Model file for the job. Use its own axes, mm. Round coordinates to 2 decimals unless told otherwise and drop trailing zeros. Order: outer loops, then holes, each group sorted by start corner. A loop starts at its lowest first (then second) coordinate and runs counter-clockwise, first axis right, second up. Notation, with made-up numbers: (-24.5, 2) -> (0.5, 2) arc R12 cw to (0.5, 7) -> close; hole circle Ø2 at (37, 63.5). An arc over 180 degrees is marked (long way). Put each result on its own line as item: value. Start each with the question number.
Q1. Cut at C-C, the plane y = -0.2. List the corners of the cut face in (x, z), and give its area (3 significant figures).
Q2. Flat gauge pins, fed straight in: P1, Ø1, axis at x = 1, y = 0.5, coming from the +Z side; P2, Ø1, axis at y = -0.5, z = 4.5, coming from the -X side; P3, Ø1, axis at y = 0, z = -3.5, coming from the +X side. Where does each tip first touch, or does it go through?
Q3. Cut at D-D, the plane z = -8.5. List the corners of the cut face in (x, y).
Q4. Cut at A-A, the plane x = 63. List the corners of the cut face in (y, z), and give its area (3 significant figures).
Q5. Cut at B-B, the plane z = 106. List the corners of the cut face in (x, y), and give its area (3 significant figures).
Q6. Probe L1, parallel to X at y = 0.6, z = -5; L2, parallel to Z at x = -77.5, y = -0.55; L3, parallel to Z at x = 0.5, y = 0.4. List the from-to ranges inside material, lowest first.
from build123d import *

# Parameters (mm, degrees)
IZIM1_W                     = 120
IZIM1_H                     = 180
Y_KSEKLIK_EKSTR_ZYON1_DEPTH = 1
Y_KSEKLIK_EKSTR_ZYON3_REACH = 252.002
IZIM4_W                     = 24
IZIM4_H                     = 2
AYNALAMA2_COPY_1_REACH      = 252.002
AYNALAMA2_COPY_1_SKETCH_W   = 24
AYNALAMA2_COPY_1_SKETCH_H   = 2
RADYUS3_R                   = 80
RADYUS4_R                   = 80
RADYUS5_R                   = 170
RADYUS6_R                   = 170


with BuildPart() as part:
    # Çizim1 → Yükseklik-Ekstrüzyon1 (new, symmetric)
    with BuildSketch(Plane(origin=(0, 0, 0), x_dir=(1, 0, 0), z_dir=(0, 1, 0))):
        Rectangle(IZIM1_W, IZIM1_H)
    extrude(amount=Y_KSEKLIK_EKSTR_ZYON1_DEPTH, both=True)

    # Çizim4 → Yükseklik-Ekstrüzyon3 (add, up to next)
    with BuildSketch(Plane(origin=(78.675049056, 0, -118.012573584), x_dir=(-0.8320502943378438, 0, -0.5547001962252289), z_dir=(0.5547001962252289, 0, -0.8320502943378438)), mode=Mode.PRIVATE) as y_kseklik_ekstr_zyon3_sk1:
        Rectangle(IZIM4_W, IZIM4_H)
    y_kseklik_ekstr_zyon3_tool1 = extrude(y_kseklik_ekstr_zyon3_sk1.sketch, amount=-Y_KSEKLIK_EKSTR_ZYON3_REACH, mode=Mode.PRIVATE) - part.part
    y_kseklik_ekstr_zyon3 = y_kseklik_ekstr_zyon3_tool1.solids().sort_by_distance((78.675049, 0, -118.012574))[0]
    add(y_kseklik_ekstr_zyon3)

    # Aynalama1: Yükseklik-Ekstrüzyon3 across plane
    add(y_kseklik_ekstr_zyon3.mirror(Plane(origin=(0, 0, 0), x_dir=(0, 0, 1), z_dir=(1, 0, 0))))

    # Aynalama2: Yükseklik-Ekstrüzyon3 across plane
    add(y_kseklik_ekstr_zyon3.mirror(Plane.XY))

    # Aynalama2 copy 1 sketch → Aynalama2 copy 1 (add, up to next)
    with BuildSketch(Plane(origin=(-78.675049056, 0, 118.012573584), x_dir=(0.8320502943378438, 0, 0.5547001962252289), z_dir=(-0.5547001962252289, 0, 0.8320502943378438)), mode=Mode.PRIVATE) as aynalama2_copy_1_sk1:
        Rectangle(AYNALAMA2_COPY_1_SKETCH_W, AYNALAMA2_COPY_1_SKETCH_H)
    aynalama2_copy_1_tool1 = extrude(aynalama2_copy_1_sk1.sketch, amount=-AYNALAMA2_COPY_1_REACH, mode=Mode.PRIVATE) - part.part
    add(aynalama2_copy_1_tool1.solids().sort_by_distance((-78.675049, 0, 118.012574))[0])

    # Radyus3
    # the kernel refuses this fillet: 80 mm, written as the material it adds along each edge
    with BuildSketch(Plane(origin=(45.577794898, 1, -90), x_dir=(-1, 0, 0), z_dir=(0, -1, 0))) as radyus3_piece_1:
        with BuildLine():
            CenterArc((42.804708678, 80), RADYUS3_R, 214.516100583, 55.483899417)
            Line((-23.112650626, 34.668975939), (-24.430997812, 33.762355458))
            ThreePointArc((-24.430997812, 33.762355458), (-12.887605784, 16.446967656), (-1.331280471, -0.887520314))
            Line((-1.331280471, -0.887520314), (0, -1.6))
            Line((0, -1.6), (42.804708678, -1.6))
            Line((42.804708678, -1.6), (42.804708678, 0))
        make_face()
    extrude(amount=2)
    with BuildSketch(Plane(origin=(-45.577794898, 1, -90), x_dir=(-0.5547001962252296, 0, -0.8320502943378434), z_dir=(0, -1, 0))) as radyus3_piece_2:
        with BuildLine():
            CenterArc((42.820243244, 79.991686152), RADYUS3_R, 213.690067526, 55.483899417)
            Line((-23.743780303, 35.615670454), (-25.075060774, 34.72815014))
            Line((-25.075060774, 34.72815014), (-1.331280471, -0.887520314))
            Line((-1.331280471, -0.887520314), (0, -1.6))
            ThreePointArc((0, -1.6), (20.833461736, -1.6), (41.643857077, -1.599833723))
            Line((41.643857077, -1.599833723), (41.666923472, 0))
        make_face()
    extrude(amount=2)

    # Radyus4
    # the kernel refuses this fillet: 80 mm, written as the material it adds along each edge
    with BuildSketch(Plane(origin=(-45.577794898, 1, 90), x_dir=(1, 0, 0), z_dir=(0, -1, 0))) as radyus4_piece_1:
        with BuildLine():
            CenterArc((42.804708678, 80), RADYUS4_R, 214.516100583, 55.483899417)
            Line((-23.112650626, 34.668975939), (-24.430997812, 33.762355458))
            ThreePointArc((-24.430997812, 33.762355458), (-12.887605784, 16.446967656), (-1.331280471, -0.887520314))
            Line((-1.331280471, -0.887520314), (0, -1.6))
            Line((0, -1.6), (42.804708678, -1.6))
            Line((42.804708678, -1.6), (42.804708678, 0))
        make_face()
    extrude(amount=2)
    with BuildSketch(Plane(origin=(45.577794898, 1, 90), x_dir=(0.5547001962252287, 0, 0.8320502943378439), z_dir=(0, -1, 0))) as radyus4_piece_2:
        with BuildLine():
            CenterArc((42.820243244, 79.991686152), RADYUS4_R, 213.690067526, 55.483899417)
            Line((-23.743780303, 35.615670454), (-25.075060774, 34.72815014))
            Line((-25.075060774, 34.72815014), (-1.331280471, -0.887520314))
            Line((-1.331280471, -0.887520314), (0, -1.6))
            ThreePointArc((0, -1.6), (20.833461736, -1.6), (41.643857077, -1.599833723))
            Line((41.643857077, -1.599833723), (41.666923472, 0))
        make_face()
    extrude(amount=2)

    # Radyus5
    radyus5_edges = [part.edges().sort_by_distance(p)[0] for p in [
        (-60, 0, -68.366692347),
        (-60, 0, 68.366692347),
    ]]
    fillet(radyus5_edges, radius=RADYUS5_R)

    # Radyus6
    radyus6_edges = [part.edges().sort_by_distance(p)[0] for p in [
        (60, 0, -68.366692347),
        (60, 0, 68.366692347),
    ]]
    fillet(radyus6_edges, radius=RADYUS6_R)


solid = part.part
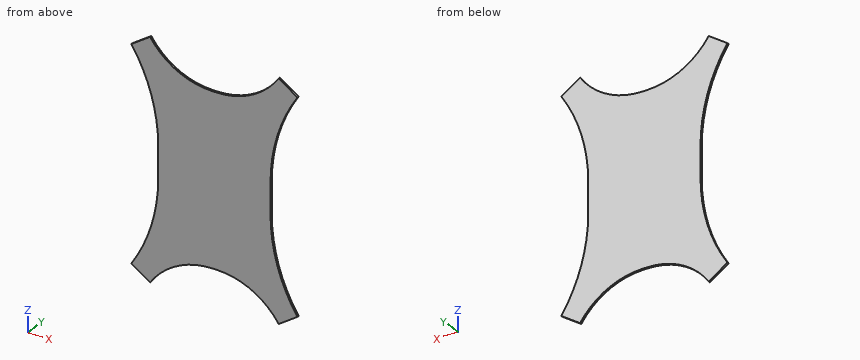
Ans:
1. outline: (-88.66, -111.36) -> (-68.69, -124.67) arc R80 cw to (-2.77, -90) -> (2.77, -90) arc R80 cw to (68.69, -124.67) -> (88.66, -111.36) -> (88.55, -111.19) arc R170 cw to (60, -16.89) -> (60, 16.89) arc R170 cw to (88.55, 111.19) -> (88.66, 111.36) -> (68.69, 124.67) arc R80 cw to (2.77, 90) -> (-2.77, 90) arc R80 cw to (-68.69, 124.67) -> (-88.66, 111.36) -> (-88.55, 111.19) arc R170 cw to (-60, 16.89) -> (-60, -16.89) arc R170 cw to (-88.55, -111.19) -> close
1. area: 27,600 mm^2
2. P1: stops at z = 90
2. P2: stops at x = -60
2. P3: stops at x = 60
3. outline: (-60, -1) -> (60, -1) -> (60, 1) -> (-60, 1) -> close
4. outline: (-1, -117.34) -> (1, -117.34) -> (1, -48.69) -> (-1, -48.69) -> close; (-1, 48.69) -> (1, 48.69) -> (1, 117.34) -> (-1, 117.34) -> close
4. area: 275 mm^2
5. outline: (-85.22, -1) -> (-50.77, -1) -> (-50.77, 1) -> (-85.22, 1) -> close; (50.77, -1) -> (85.22, -1) -> (85.22, 1) -> (50.77, 1) -> close
5. area: 138 mm^2
6. L1: x = -60 to 60
6. L2: z = -118.8 to -92.02, 92.02 to 118.8
6. L3: z = -90 to 90
